from build123d import *

# Parameters (mm, degrees)
BOSS_EXTRUDE1_DEPTH = 14
BOSS_EXTRUDE2_DEPTH = 2
BOSS_EXTRUDE3_DEPTH = 2
SKETCH4_R           = 2.125
CUT_EXTRUDE1_DEPTH  = 15
SKETCH5_R           = 1.6
CUT_EXTRUDE2_DEPTH  = 15
SKETCH6_W           = 7
SKETCH6_H           = 6
CUT_EXTRUDE3_DEPTH  = 15
SKETCH7_W           = 7
SKETCH7_H           = 6
CUT_EXTRUDE4_DEPTH  = 15
FILLET2_R           = 10
FILLET3_R           = 10


with BuildPart() as part:
    # Sketch1 → Boss-Extrude1 (new body)
    with BuildSketch(Plane(origin=(0, 0, 0), x_dir=(1, 0, 0), z_dir=(0, 1, 0))):
        Polygon((-27.184182145, 10), (2.815817855, 10), (24.029021291, -11.213203436), (22.614807728, -12.627416998), (1.98739073, 8), (-27.184182145, 8), align=None)
    extrude(amount=BOSS_EXTRUDE1_DEPTH)

    # Sketch2 → Boss-Extrude2 (add)
    with BuildSketch(Plane(origin=(0, 14, 0), x_dir=(1, 0, 0), z_dir=(0, 1, 0))):
        Polygon((-27.184182145, 8), (-27.184182145, -2), (-2.154744893, -2), (15.543739917, -19.69848481), (22.614807728, -12.627416998), (1.98739073, 8), align=None)
    extrude(amount=-BOSS_EXTRUDE2_DEPTH)

    # Sketch3 → Boss-Extrude3 (add)
    with BuildSketch(Plane.XZ):
        Polygon((-27.184182145, -8), (-27.184182145, 2), (-2.154744893, 2), (15.543739917, 19.69848481), (22.614807728, 12.627416998), (1.98739073, -8), align=None)
    extrude(amount=-BOSS_EXTRUDE3_DEPTH)

    # Sketch4 → Cut-Extrude1 (cut)
    with BuildSketch(Plane(origin=(0, 14, 0), x_dir=(1, 0, 0), z_dir=(0, 1, 0))):
        with Locations(Location((-21.184182145, 3, 0), (0, 0, 270))):
            Circle(SKETCH4_R)
        with Locations(Location((-11.184182145, 3, 0), (0, 0, 270))):
            Circle(SKETCH4_R)
        with Locations(Location((7.765565323, -4.849242405, 0), (0, 0, 270))):
            Circle(SKETCH4_R)
        with Locations(Location((14.836633135, -11.920310217, 0), (0, 0, 270))):
            Circle(SKETCH4_R)
    extrude(amount=-CUT_EXTRUDE1_DEPTH, mode=Mode.SUBTRACT)

    # Sketch5 → Cut-Extrude2 (cut)
    with BuildSketch(Plane(origin=(0, 14, 0), x_dir=(1, 0, 0), z_dir=(0, 1, 0))):
        with Locations(Location((1.667767558, 7.228361402, 0), (0, 0, 270))):
            Circle(SKETCH5_R)
    extrude(amount=-CUT_EXTRUDE2_DEPTH, mode=Mode.SUBTRACT)

    # Sketch6 → Cut-Extrude3 (cut)
    with BuildSketch(Plane(origin=(0, 0, -10), x_dir=(-1, 0, 0), z_dir=(0, 0, -1))):
        with Locations((0.684182145, 7)):
            Rectangle(SKETCH6_W, SKETCH6_H)
    extrude(amount=-CUT_EXTRUDE3_DEPTH, mode=Mode.SUBTRACT)

    # Sketch7 → Cut-Extrude4 (cut)
    with BuildSketch(Plane(origin=(6.407908928, 0, -6.407908928), x_dir=(-0.7071067811865465, 0, -0.7071067811865487), z_dir=(0.7071067811865487, 0, -0.7071067811865465))):
        with Locations((1.579983912, 7)):
            Rectangle(SKETCH7_W, SKETCH7_H)
    extrude(amount=-CUT_EXTRUDE4_DEPTH, mode=Mode.SUBTRACT)

    # Fillet2
    fillet2_edges = [part.edges().sort_by_distance(p)[0] for p in [
        (2.815817855, 2, -10),
        (2.815817855, 12, -10),
    ]]
    fillet(fillet2_edges, radius=FILLET2_R)

    # Fillet3
    fillet3_edges = [part.edges().sort_by_distance(p)[0] for p in [
        (-2.154744893, 13, 2),
        (-2.154744893, 1, 2),
    ]]
    fillet(fillet3_edges, radius=FILLET3_R)


solid = part.part
Here's how the part is built. I have some questions about the finished solid (model axes, mm). A direction names the side the tool comes from. Round coordinates to 2 decimals unless told otherwise and drop trailing zeros. Order: outer loops, then holes, each group sorted by start corner. A loop starts at its lowest first (then second) coordinate and runs counter-clockwise, first axis right, second up. Notation, with made-up numbers: (70, 81) -> (106, 81) arc R30 cw to (106, 109) -> close; hole circle Ø1 at (54.25, 87). An arc over 180 degrees is marked (long way). Use CSV: the item, a comma, the result in double quotes.
1. I want a section at D-D on z = -3. List the corners of the cut face in (x, y) for me, and give its area (3 significant figures).
Recorded:
outline,"(-27.18, 0) -> (-23.31, 0) -> (-23.31, 2) -> (-27.18, 2) -> close; (-27.18, 12) -> (-23.31, 12) -> (-23.31, 14) -> (-27.18, 14) -> close; (-19.06, 0) -> (-13.31, 0) -> (-13.31, 2) -> (-19.06, 2) -> close; (-19.06, 12) -> (-13.31, 12) -> (-13.31, 14) -> (-19.06, 14) -> close; (-9.06, 0) -> (9.82, 0) -> (9.82, 14) -> (-9.06, 14) -> (-9.06, 12) -> (6.99, 12) -> (6.99, 2) -> (-9.06, 2) -> close"
area,"142 mm2"
2. I want a section at A-A on x = 8.5. List the corners of the cut face in (y, z) for me, and give its area (3 significant figures).
Recorded:
outline,"(0, -4.32) -> (14, -4.32) -> (14, 2.86) -> (12, 2.86) -> (12, -1.49) -> (2, -1.49) -> (2, 2.86) -> (0, 2.86) -> close; (0, 6.84) -> (2, 6.84) -> (2, 12.65) -> (0, 12.65) -> close; (12, 6.84) -> (14, 6.84) -> (14, 12.65) -> (12, 12.65) -> close"
area,"80.2 mm2"
3. I want a section at B-B on z = 6. List the corners of the cut face in (x, y) for me, and give its area (3 significant figures).
Recorded:
outline,"(1.85, 0) -> (5.98, 0) -> (5.98, 2) -> (1.85, 2) -> close; (1.85, 12) -> (5.98, 12) -> (5.98, 14) -> (1.85, 14) -> close; (9.55, 0) -> (18.82, 0) -> (18.82, 14) -> (9.55, 14) -> (9.55, 12) -> (15.99, 12) -> (15.99, 2) -> (9.55, 2) -> close"
area,"81.9 mm2"
4. Which directions (+Z, -Z, +X, -X, +Y, -Y) give clear straight access to the entire face, cutting with the end or side of a thin tool? Please do faces 4 (the face through (2.55, 2.03, -9.22)), 5 (the face through (-19.75, 1.01, -4.57)), 6 (the face through (-4.184, 7, -9)), 7 (the face through (7.068, 6.958, -4.353)), 8 (the face through (-2, 12, 1)).
Recorded:
face 4,"-Z, +X, +Y, -Y"
face 5,"+Y, -Y"
face 6,"+Z, -Z, +X"
face 7,"-Z, -X"
face 8,"+Z, -X"
5. I need wall thicknesses on line 1 along Y through (x, z) = (0, -0.75); line 2 along Z through (x, y) = (15, 0.5); line 3 along Z through (x, y) = (-5.5, 3.25). Which ranges of each line are inside material? Lowest first, please.
Recorded:
line 1,"y = 0 to 2, 12 to 14"
line 2,"z = 2.18 to 9.8, 14.04 to 19.15"
line 3,"z = -10 to -8"
6. I'm going to push flat-ended pins straight in: P1, Ø1.5, axis at x = 2.5, y = 7.5, coming from the +Z side; P2, Ø7, axis at x = -21.18, z = -3, coming from the -Y side; P3, Ø5, axis at x = -7.5, y = 8, coming from the +Z side; P4, Ø1, axis at x = 14.5, y = 3.5, coming from the -Z side. Where does each tip first touch, or does it pass through?
Recorded:
P1,"passes through"
P2,"stops at y = 0"
P3,"stops at z = -8"
P4,"stops at z = 1.18"
7. I want a section at C-C on y = 8.25. List the corners of the cut face in (x, z) for me.
Recorded:
outline,"(-27.18, -10) -> (-4.18, -10) -> (-4.18, -8) -> (-27.18, -8) -> close; (6.35, -3.64) -> (7.77, -5.05) -> (24.03, 11.21) -> (22.61, 12.63) -> close"
8. Thinking about a two-plate mould opening in Z: for faces 1 (the face through (-9.75, 1.01, -4.57)), 2 (the face through (2, 10, -9)), 3 (the face through (-14, 7, -10)), which applies, pulls with the +Z half, pulls with the -Z half, needs draft (parallel to the pull), parting line crosses it, or undercut?
Recorded:
face 1,"undercut"
face 2,"needs draft"
face 3,"pulls with the -Z half"
